Build history of the part. All positions in model axes, mm. A direction names the side the tool comes from. Give positions to 0.01 mm unless a question says otherwise; leave off trailing zeros. Loops run counter-clockwise (first coordinate to the right, second up) from the corner with the lowest first, then second, coordinate; pieces in that order, holes last. Notation, with made-up numbers: (-38.5, -4.75) -> (6.5, -4.75) arc R25 cw to (6.5, 14.25) -> close; hole circle Ø3 at (73, 71). An arc over 180 degrees is marked (long way). Answer as a JSON object with one key per item and string values. Group by question number.
Q1. Band-saw the part on C-C, the plane x = -516. Write the cut outline in (y, z), plus the area to 3 significant figures.
Q2. Two-plate mould, pull along Z, no slides. Class faces 1 (the flat face through (-454, 249, 5)), 2 (the flat face through (-454, 245, 10)), 3 (the cylindrical face through (-335.08, 244.08, 9.49)): pulls with the +Z half, pulls with the -Z half, needs draft (parallel to the pull), parting line crosses it, or undercut.
Q3. Tool access for faces 4 (the flat face through (-332.295, 249.4, 4.9)), 5 (the flat face through (-454, 245, 9)): list every direction of +Z, -Z, +X, -X, +Y, -Y with a clear straight run to the whole face (end or side of a thin tool).
Q4. Drop a flat-ended pin along its axis: pin 1 (4 mm diameter, centred on x = -567.29, y = 245, fed in from -Z). Give the stop position or say it passes through.
Q5. Band-saw the part on B-B, the plane z = 7.5. Write the cut outline in (x, y).
Q6. Wall check: probe 1 along X at (y, z) = (245, 0.6); probe 2 along Z at (x, y) = (-434.5, 245.25); probe 3 along Y at (x, z) = (-417.5, 5.25). Give the ranges that are in metal, low to high. Write a range as from..to.
Q7. Band-saw the part on A-A, the plane y = 245. Count the separate pieces of the cut face and the enclosed holes in it, plus the area to 3 significant figures.
from build123d import *

# Parameters (mm, degrees)
SKETCH_1_W          = 240
SKETCH_1_H          = 10
SKETCH_1_R          = 1.6
SKETCH_1_R_2        = 2.4
EXTRUDE_1_DEPTH     = 10
SKETCH_2_W          = 8
SKETCH_2_H          = 8
CUT_EXTRUDE_1_DEPTH = 347.698716467


with BuildPart() as part:
    # ｽｹｯﾁ1 → ﾎﾞｽ - 押し出し1 (new body)
    with BuildSketch(Plane.XY):
        with Locations((-452.2947342, 245)):
            Rectangle(SKETCH_1_W, SKETCH_1_H)
        with Locations((-567.2947342, 244.999999998)):
            Circle(SKETCH_1_R, mode=Mode.SUBTRACT)
        with Locations((-547.2947342, 244.999999998)):
            Circle(SKETCH_1_R, mode=Mode.SUBTRACT)
        with Locations((-337.2947342, 245)):
            Circle(SKETCH_1_R_2, mode=Mode.SUBTRACT)
    extrude(amount=EXTRUDE_1_DEPTH)

    # ｽｹｯﾁ2 → ｶｯﾄ - 押し出し1 (cut, through all)
    with BuildSketch(Plane.ZY.offset(572.2947342)):
        with Locations((5, 245)):
            Rectangle(SKETCH_2_W, SKETCH_2_H)
    extrude(amount=-CUT_EXTRUDE_1_DEPTH, mode=Mode.SUBTRACT)


solid = part.part
Worked answers:
{
 "1": {"outline": "(240, 0) -> (250, 0) -> (250, 10) -> (240, 10) -> close; hole (241, 1) -> (249, 1) -> (249, 9) -> (241, 9) -> close", "area": "36.0 mm2"},
 "2": {"face 1": "undercut", "face 2": "pulls with the +Z half", "face 3": "needs draft"},
 "3": {"face 4": "+Z, -Z, +X, +Y, -Y", "face 5": "+X, -X"},
 "4": {"pin 1": "z = 0"},
 "5": {"outline": "(-572.29, 240) -> (-332.29, 240) -> (-332.29, 241) -> (-572.29, 241) -> close; (-572.29, 249) -> (-332.29, 249) -> (-332.29, 250) -> (-572.29, 250) -> close"},
 "6": {"probe 1": "-572.29..-568.89, -565.69..-548.89, -545.69..-339.69, -334.89..-332.29", "probe 2": "0..1, 9..10", "probe 3": "240..241, 249..250"},
 "7": {"separate pieces": "8", "enclosed holes": "0", "area": "458 mm2"}
}
